Input: part model. Units: mm. Frame: model coordinates. A direction names the side the tool comes from. Round coordinates to 2 decimals unless told otherwise and drop trailing zeros. Order: outer loops, then holes, each group sorted by start corner. A loop starts at its lowest first (then second) coordinate and runs counter-clockwise, first axis right, second up. Notation, with made-up numbers: M -9.75,3.5 L -0.75,3.5 A27 ccw -0.75,20.5 Z; hole C -14,31.5 d11. An arc over 180 degrees is marked long. One line per question, with ' | ' between items.
```python
from build123d import *

# Parameters (mm, degrees)
EXTRUDE_1_DEPTH     = 30
SKETCH_2_W          = 9
SKETCH_2_H          = 14
CUT_EXTRUDE_1_DEPTH = 15
SKETCH_3_R          = 2
CUT_EXTRUDE_2_DEPTH = 32


with BuildPart() as part:
    # 草图1 → 凸台-拉伸1 (new body)
    with BuildSketch(Plane.XY):
        with BuildLine():
            Line((4, 0), (20, 0))
            Line((20, 0), (20, -4))
            Line((20, -4), (0, -4))
            ThreePointArc((0, -4), (-2.828427125, 2.828427125), (4, 0))
        make_face()
    extrude(amount=EXTRUDE_1_DEPTH)

    # 草图2 → 切除-拉伸1 (cut)
    with BuildSketch(Plane.XZ.offset(4)):
        with Locations((0, 15)):
            Rectangle(SKETCH_2_W, SKETCH_2_H)
    extrude(amount=-CUT_EXTRUDE_1_DEPTH, mode=Mode.SUBTRACT)

    # 草图3 → 切除-拉伸2 (cut)
    with BuildSketch(Plane(origin=(0, 0, 0), x_dir=(-1, 0, 0), z_dir=(0, 0, -1))):
        with Locations(Location((0, 0, 0), (0, 0, 180))):
            Circle(SKETCH_3_R)
    extrude(amount=-CUT_EXTRUDE_2_DEPTH, mode=Mode.SUBTRACT)


solid = part.part
```
Item 1: Line query: line 1 along Y through (x, z) = (0, 24.5); line 2 along Z through (x, y) = (-0.75, 3.75); line 3 along Y through (x, z) = (17.5, 6.75). Output: solid intervals per line, ascending. Write a range as from..to.
Report:
line 1: -4..-2, 2..4 | line 2: 0..8, 22..30 | line 3: -4..0
Item 2: Access query for faces 5 (the flat face through (8, -1, 0)), 6 (the flat face through (4.5, -2, 15)), 7 (the flat face through (12, 0, 15)). Directions: +Z, -Z, +X, -X, +Y, -Y. A direction counts if a zero-diameter tool reaches every point of the face in a straight line with its end or side. Return the directions, or none.
Report:
face 5: -Z, +X, -X, +Y, -Y | face 6: -X, +Y, -Y | face 7: +Z, -Z, +X, +Y
Item 3: Section query A-A, the plane z = 4.75. Return loops of the section in (x, y).
Report:
outline: M 0,-4 L 20,-4 L 20,0 L 4,0 A4 ccw long Z; hole C 0,0 d4
Item 4: Section query D-D, the plane x = 3. Return loops of the section in (y, z).
Report:
outline: M -4,0 L 2.65,0 L 2.65,8 L -4,8 Z; M -4,22 L 2.65,22 L 2.65,30 L -4,30 Z
Item 5: First-contact query: pin 1 (1.2 mm diameter, centred on y = -1.5, z = 15.5, fed in from -X); pin 2 (2 mm diameter, centred on y = 2.5, z = 7, fed in from +X); pin 3 (3.5 mm diameter, centred on x = 0, y = 0, fed in from -Z). Flat tips, straight axial feed; report the tip coordinate or a pass-through.
Report:
pin 1: x = 4.5 | pin 2: x = 3.71 | pin 3: through
Item 6: Section query B-B, the plane x = 0.5. Return loops of the section in (y, z).
Report:
outline: M -4,0 L -1.94,0 L -1.94,8 L -4,8 Z; M -4,22 L -1.94,22 L -1.94,30 L -4,30 Z; M 1.94,0 L 3.97,0 L 3.97,8 L 1.94,8 Z; M 1.94,22 L 3.97,22 L 3.97,30 L 1.94,30 Z
Item 7: Mould query, pull axis X, two halves, no side actions, for faces 1 (the flat face through (20, -2, 15)), 2 (the cylindrical face through (0, 2, 26)), 3 (the flat face through (1, -2, 8)), 4 (the cylindrical face through (-2.92, 2.734, 3.944)). Classes: +X half, -X half, draft (parallel to the pull), parting line (faces both ways), or undercut.
Report:
face 1: +X half | face 2: undercut | face 3: draft | face 4: parting line
Item 8: Section query C-C, the plane y = 1. Return loops of the section in (x, z), plus the area to 3 significant figures.
Report:
outline: M -3.87,0 L -1.73,0 L -1.73,8 L -3.87,8 Z; M -3.87,22 L -1.73,22 L -1.73,30 L -3.87,30 Z; M 1.73,0 L 3.87,0 L 3.87,8 L 1.73,8 Z; M 1.73,22 L 3.87,22 L 3.87,30 L 1.73,30 Z | area: 68.5 mm²
